Model file for the job. Use its own axes, mm. A direction names the side the tool comes from. Give positions to 0.01 mm unless a question says otherwise; leave off trailing zeros. Write each loop counter-clockwise with the first axis right and the second up, starting at its lowest first coordinate (ties: lowest second). Pieces come first, ordered by that corner, then holes.
```python
from build123d import *

# Parameters (mm, degrees)
F0_W     = 53.322375752
F0_H     = 50.9416181594
F1_DEPTH = 52.578
F2_W     = 9.497590363
F2_H     = 5.180504173
F2_W_2   = 4.0292814374
F2_H_2   = 23.3122664504
F3_DEPTH = 2.54


with BuildPart() as f1:
    # F0 (on Top) → F1 (new body)
    with BuildSketch(Plane.XY):
        with Locations((-49.3195350282, 50.2221053466)):
            Rectangle(F0_W, F0_H)
    extrude(amount=F1_DEPTH)

    # F2 (on face) → F3 (join)
    with BuildSketch(Plane.XZ.offset(-24.7512962669)):
        with Locations((-56.8416379392, 32.5220506638)):
            Rectangle(F2_W, F2_H)
        Polygon((-48.0635613203, 35.1980318357), (-52.0928427577, 35.1123027503), (-52.0928427577, 29.9317985773), (-48.0635613203, 29.9317985773), align=None)
        Polygon((-38.5659709573, 35.4001075029), (-48.0635613203, 35.1980318357), (-48.0635613203, 29.9317985773), (-38.5659709573, 29.9317985773), align=None)
        with Locations((-50.078202039, 18.2756653521)):
            Rectangle(F2_W_2, F2_H_2)
        Polygon((-48.0635613203, 47.7757565677), (-52.0928427577, 47.7757565677), (-52.0928427577, 35.1123027503), (-48.0635613203, 35.1980318357), align=None)
    extrude(amount=F3_DEPTH)


solid = f1.part
```
1. Pin check, flat tips, straight feed: P1, Ø3, axis at x = -41.5, y = 24, coming from the -Z side; P2, Ø0.8, axis at x = -56, y = 23, coming from the -Z side; P3, Ø1.3, axis at x = -58, y = 24, coming from the +Z side; P4, Ø2, axis at x = -69.5, z = 30.5, coming from the -Y side. Stop position of each tip, or through.
Calculated:
P1: stops at z = 0
P2: stops at z = 29.93
P3: stops at z = 35.11
P4: stops at y = 24.75
2. Slice it at C-C, the plane x = -30.5. Write the cut outline in (y, z), and give its area (3 significant figures).
Calculated:
outline: (24.75, 0) - (75.69, 0) - (75.69, 52.58) - (24.75, 52.58) - close
area: 2,680 mm2
3. Slice it at B-B, the plane z = 16. Write the cut outline in (x, y).
Calculated:
outline: (-75.98, 24.75) - (-52.09, 24.75) - (-52.09, 22.21) - (-48.06, 22.21) - (-48.06, 24.75) - (-22.66, 24.75) - (-22.66, 75.69) - (-75.98, 75.69) - close
4. Slice it at A-A, the plane x = -57. Write the cut outline in (y, z).
Calculated:
outline: (22.21, 29.93) - (24.75, 29.93) - (24.75, 0) - (75.69, 0) - (75.69, 52.58) - (24.75, 52.58) - (24.75, 35.11) - (22.21, 35.11) - close
5. Probe probe 1 along Y at (x, z) = (-56, 22.5). List the from-to ranges inside material, lowest first.
Calculated:
probe 1: y = 24.75 to 75.69
6. Which spindle directions (+Z, -Z, +X, -X, +Y, -Y) get a long thin tool onto all of the face, cutting with end or side? Do faces 1 (the flat face through (-57, 23, 29.932)), 2 (the flat face through (-50, 23, 6.62)), 3 (the flat face through (-43, 23, 29.932)), 4 (the flat face through (-61.59, 23, 32)). Say none if no direction does.
Calculated:
face 1: -Z, -X, -Y
face 2: -Z, +X, -X, -Y
face 3: -Z, +X, -Y
face 4: +Z, -Z, -X, -Y
